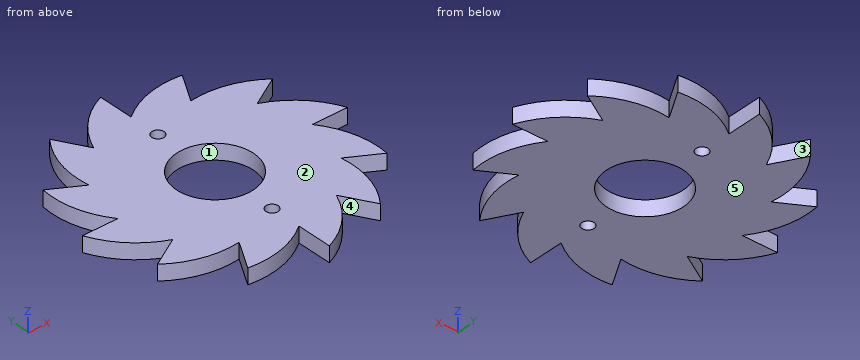
```python
from build123d import *

# Parameters (mm, degrees)
SKETCH1_R           = 38.1
SKETCH1_R_2         = 1.7526
SKETCH1_R_3         = 10.9982
BOSS_EXTRUDE1_DEPTH = 4.445
CUT_EXTRUDE1_DEPTH  = 55.064572735
CIRPATTERN1_COUNT   = 12


with BuildPart() as part:
    # Sketch1 → Boss-Extrude1 (new body)
    with BuildSketch(Plane.XY):
        Circle(SKETCH1_R)
        with Locations((0, 18.9992)):
            Circle(SKETCH1_R_2, mode=Mode.SUBTRACT)
        Circle(SKETCH1_R_3, mode=Mode.SUBTRACT)
        with Locations((0, -18.9992)):
            Circle(SKETCH1_R_2, mode=Mode.SUBTRACT)
    extrude(amount=BOSS_EXTRUDE1_DEPTH)

    # Sketch3 → Cut-Extrude1 (cut, through all)
    with BuildSketch(Plane.XY.offset(4.445)):
        with BuildLine():
            Line((-19.05, 32.995567884), (-13.97, 24.196749782))
            ThreePointArc((-13.97, 24.196749782), (-8.388518849, 32.558632061), (0, 38.1))
            ThreePointArc((0, 38.1), (-9.861005618, 36.801773982), (-19.05, 32.995567884))
        make_face()
    cut_extrude1 = extrude(amount=-CUT_EXTRUDE1_DEPTH, mode=Mode.SUBTRACT)

    # CirPattern1: Cut-Extrude1 ×12 about axis
    cirpattern1_axis = Axis((0, 0, 0), (0, 0, 1))
    for i in range(1, CIRPATTERN1_COUNT):
        add(cut_extrude1.rotate(cirpattern1_axis, i * 360 / CIRPATTERN1_COUNT), mode=Mode.SUBTRACT)


solid = part.part
```
Part model, mm, in its own coordinate system. Face numbers are marked on the shaded views. A direction names the side the tool comes from. Round coordinates to 2 decimals unless told otherwise and drop trailing zeros. Loops run counter-clockwise (first coordinate to the right, second up) from the corner with the lowest first, then second, coordinate; pieces in that order, holes last.
Item 1: Drill centre lines: line 1 (X direction, y = -30, z = 1.4); line 2 (Y direction, x = 30.5, z = 3.25); line 3 (X direction, y = 31, z = 1.65). Where is each one in solid material? Low to high.
Item 2: Cut at B-B, the plane z = 0.9. Give the cut face in (x, y), then the cut area to 3 significant figures.
Item 3: 3-axis set-ups, long thin cutter, end or side, ignore diameter. For the marked faces 3, 4 and 5: which of +Z, -Z, +X, -X, +Y, -Y reach the whole face in a straight line?
Item 4: Drop flat-ended pins along their axis: P1, Ø1.3, axis at x = -35, z = 1.5, coming from the +Y side; P2, Ø2, axis at x = 13, z = 3.5, coming from the -Y side; P3, Ø1.5, axis at y = 11.5, z = 1, coming from the -X side. Give the stop position or say it passes through.
Item 5: Cut at D-D, the plane y = 23. Give the cut face in (x, z) (3 decimals), then the cut area to 3 significant figures.
Item 6: Mould opens along X. For the marked faces 1 and 2 say: +X half, -X half, draft (parallel to the pull), parting line (faces both ways), or undercut.
Item 7: Cut at A-A, the plane y = -7.5. Give the cut face in (x, z) (3 decimals), then the cut area to 3 significant figures.
Item 8: Cut at C-C, the plane y = -27. Give the cut face in (x, z) (3 decimals), then the cut area to 3 significant figures.
A:
1. line 1: x = -17.32 to -3.12, 0 to 10.64, 17.32 to 21.06
1. line 2: y = -17.61 to -4.05, 0 to 10.24, 17.61 to 20.77
1. line 3: x = -20.46 to -17.9, -9.83 to 0, 5.1 to 17.9
2. outline: (-38.1, 0) arc R25.4 ccw to (-24.2, -13.97) - (-33, -19.05) arc R25.4 ccw to (-13.97, -24.2) - (-19.05, -33) arc R25.4 ccw to (0, -27.94) - (0, -38.1) arc R25.4 ccw to (13.97, -24.2) - (19.05, -33) arc R25.4 ccw to (24.2, -13.97) - (33, -19.05) arc R25.4 ccw to (27.94, 0) - (38.1, 0) arc R25.4 ccw to (24.2, 13.97) - (33, 19.05) arc R25.4 ccw to (13.97, 24.2) - (19.05, 33) arc R25.4 ccw to (0, 27.94) - (0, 38.1) arc R25.4 ccw to (-13.97, 24.2) - (-19.05, 33) arc R25.4 ccw to (-24.2, 13.97) - (-33, 19.05) arc R25.4 ccw to (-27.94, 0) - close; hole circle Ø22 at (0, 0); hole circle Ø3.51 at (0, -19); hole circle Ø3.51 at (0, 19)
2. area: 3,110 mm2
3. face 3: +Z, -Z, +Y
3. face 4: +Z, -Z, -Y
3. face 5: -Z, +X, -X, +Y, -Y
4. P1: stops at y = 0
4. P2: stops at y = -28.03
4. P3: stops at x = -33.03
5. outline: (-23.793, 0) - (25.758, 0) - (25.758, 4.445) - (-23.793, 4.445) - close
5. area: 220 mm2
6. face 1: undercut
6. face 2: draft
7. outline: (-33.401, 0) - (-8.044, 0) - (-8.044, 4.445) - (-33.401, 4.445) - close; (8.044, 0) - (31.938, 0) - (31.938, 4.445) - (8.044, 4.445) - close
7. area: 219 mm2
8. outline: (-15.588, 0) - (12.613, 0) - (12.613, 4.445) - (-15.588, 4.445) - close; (15.588, 0) - (22.529, 0) - (22.529, 4.445) - (15.588, 4.445) - close
8. area: 156 mm2
